Input: dimensioned drawing with shaded views. Units: mm. Origin: part minimum x, y, z. Coordinates: 2 decimals unless noted, no trailing zeros. Order: outer loops, then holes, each group sorted by start corner. A loop starts at its lowest first (then second) coordinate and runs counter-clockwise, first axis right, second up. Notation, with made-up numbers: M 34.25,18.5 L 91.25,18.5 A15 cw 91.25,22.5 Z; hole C 66,61.5 d1. An arc over 180 degrees is marked long. Write item = value, one per line.
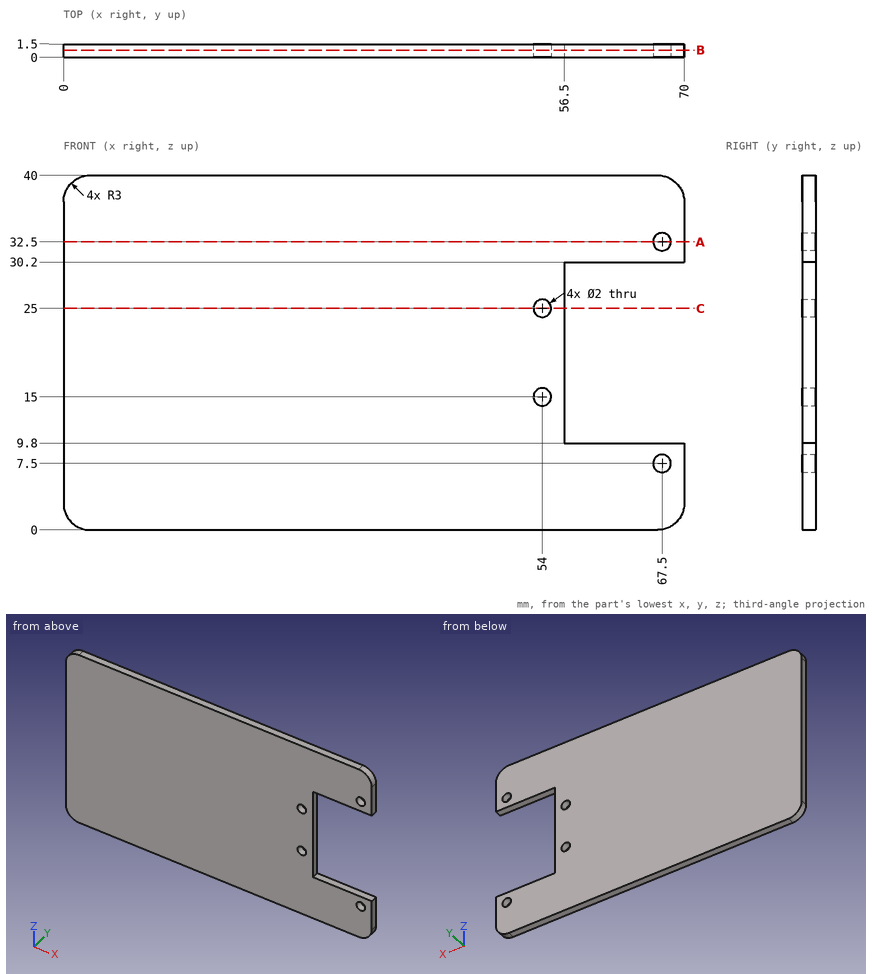
1) Section C-C, the plane z = 25. Return loops of the section in (x, y).
Numbers:
outline = M 0,0 L 53,0 L 53,1.5 L 0,1.5 Z; M 55,0 L 56.5,0 L 56.5,1.5 L 55,1.5 Z
2) Line query: L1, parallel to X at y = 0.6, z = 32.5; L2, parallel to Z at x = 65.5, y = 0.55; L3, parallel to X at y = 0.4, z = 15. Output: solid intervals per line, ascending.
Numbers:
L1 = 0 to 66.5, 68.5 to 70
L2 = 0 to 9.8, 30.2 to 40
L3 = 0 to 53, 55 to 56.5
3) Pin query (flat end, axial travel): pin 1 (1.8 mm diameter, centred on x = 67.5, z = 32.5, fed in from +Y). Return the tip coordinate at first contact, or that it passes through.
Numbers:
pin_1 = through
4) Section A-A, the plane z = 32.5. Return loops of the section in (x, y).
Numbers:
outline = M 0,0 L 66.5,0 L 66.5,1.5 L 0,1.5 Z; M 68.5,0 L 70,0 L 70,1.5 L 68.5,1.5 Z
5) Section B-B, the plane y = 0.8. Return loops of the section in (x, z).
Numbers:
outline = M 0,3 A3 ccw 3,0 L 67,0 A3 ccw 70,3 L 70,9.8 L 56.5,9.8 L 56.5,30.2 L 70,30.2 L 70,37 A3 ccw 67,40 L 3,40 A3 ccw 0,37 Z; hole C 54,15 d2; hole C 54,25 d2; hole C 67.5,7.5 d2; hole C 67.5,32.5 d2
